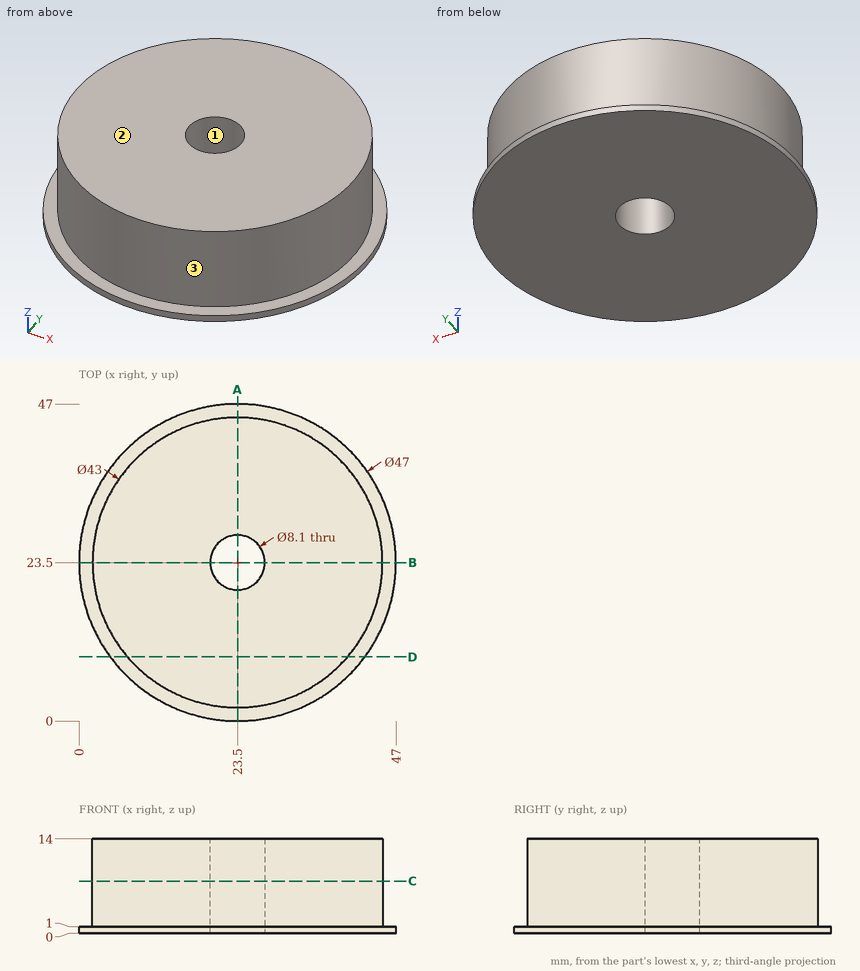
Here's the drawing with two shaded views (mm, measured from the low corner). I have some questions. Round coordinates to 2 decimals unless told otherwise and drop trailing zeros. Write each loop counter-clockwise with the first axis right and the second up, starting at its lowest first coordinate (ties: lowest second). Pieces come first, ordered by that corner, then holes. Notation, with made-up numbers: M 76.25,-18 L 134.25,-18 A3 cw 134.25,-14 Z; hole C -23.5,40 d8. An arc over 180 degrees is marked long. Answer in a Markdown table with one row per item. Add a question column.
Q1. If I drill on line 1 (Y direction, x = 23.5, z = 11); line 2 (Z direction, x = 37, y = 6.5); line 3 (Y direction, x = 25, z = 4.5), over which ranges is the centre line in solid material (lowest first)? Write a range as from..to.
Q2. Imagine slicing it at C-C (z = 7.75). Please give me the cut outline in (x, y).
Q3. If we mould it in two halves opening along X, with no side actions, what happens to the marked faces 1, 2 and 3? For each: +X half, -X half, draft (parallel to the pull), parting line (faces both ways), or undercut.
Q4. Imagine slicing it at A-A (x = 23.5). Please give me the cut outline in (y, z).
Q5. Will these pins go through, and if not, where does the flat tip stop? pin 1 Ø1.5 at (y, z) = (12.5, 7.5) entering from -X; pin 2 Ø6 at (x, z) = (14.5, 3.5) entering from -Y.
Q6. Imagine slicing it at D-D (y = 9.5). Please give me the cut outline in (x, z).
Values:
| question | item | result |
|---|---|---|
| 1 | line 1 | 2..19.45, 27.55..45 |
| 1 | line 2 | 0..1 |
| 1 | line 3 | 2.05..19.74, 27.26..44.95 |
| 2 | outline | C 23.5,23.5 d43; hole C 23.5,23.5 d8.1 |
| 3 | face 1 | undercut |
| 3 | face 2 | draft |
| 3 | face 3 | parting line |
| 4 | outline | M 0,0 L 19.45,0 L 19.45,14 L 2,14 L 2,1 L 0,1 Z; M 27.55,0 L 47,0 L 47,1 L 45,1 L 45,14 L 27.55,14 Z |
| 5 | pin 1 | x = 4.6 |
| 5 | pin 2 | y = 1.18 |
| 6 | outline | M 4.63,0 L 42.37,0 L 42.37,1 L 39.82,1 L 39.82,14 L 7.18,14 L 7.18,1 L 4.63,1 Z |
